Read the model definition and answer for the solid it produces. Units are mm, in the model's axes. A direction names the side the tool comes from. Round coordinates to 2 decimals unless told otherwise and drop trailing zeros. Loops run counter-clockwise (first coordinate to the right, second up) from the corner with the lowest first, then second, coordinate; pieces in that order, holes last. Notation, with made-up numbers: M 37.25,-11.75 L 84.25,-11.75 A22 cw 84.25,6.25 Z; hole C 65,-39.5 d8. An arc over 180 degrees is marked long. Answer as CSV lines item,"result".
```python
from build123d import *

# Parameters (mm, degrees)
SKETCH_1_W          = 60
SKETCH_1_H          = 40
SKETCH_1_R          = 8
EXTRUDE_1_DEPTH     = 3
EXTRUDE_2_DEPTH     = 3
SKETCH_6_W          = 3
SKETCH_6_H          = 68.008301529
EXTRUDE_3_DEPTH     = 60
SKETCH_7_R          = 2.5
CUT_EXTRUDE_1_DEPTH = 121.443081137
FILLET_1_R          = 10
FILLET_2_R          = 20
FILLET_4_R          = 10
FILLET_12_R         = 0.5
FILLET_13_R         = 0.5
SKETCH_10_W         = 25
SKETCH_10_H         = 2.5
EXTRUDE_6_DEPTH     = 75
FILLET_16_R         = 10


with BuildPart() as part:
    # 草图1 → 凸台-拉伸1 (new body)
    with BuildSketch(Plane(origin=(0, 0, 0), x_dir=(1, 0, 0), z_dir=(0, 1, 0))):
        with Locations((-43.647943628, 33.126585816)):
            Rectangle(SKETCH_1_W, SKETCH_1_H)
        with Locations(Location((-33.647943628, 33.126585816, 0), (0, 0, 270))):
            Circle(SKETCH_1_R, mode=Mode.SUBTRACT)
        with BuildLine():
            Line((-18.647943628, 31.626585816), (-22.647943628, 31.626585816))
            ThreePointArc((-22.647943628, 31.626585816), (-24.147943628, 33.126585816), (-22.647943628, 34.626585816))
            Line((-22.647943628, 34.626585816), (-18.647943628, 34.626585816))
            ThreePointArc((-18.647943628, 34.626585816), (-17.147943628, 33.126585816), (-18.647943628, 31.626585816))
        make_face(mode=Mode.SUBTRACT)
        with BuildLine():
            Line((-35.147943628, 18.126585816), (-35.147943628, 22.126585816))
            ThreePointArc((-35.147943628, 22.126585816), (-33.647943628, 23.626585816), (-32.147943628, 22.126585816))
            Line((-32.147943628, 22.126585816), (-32.147943628, 18.126585816))
            ThreePointArc((-32.147943628, 18.126585816), (-33.647943628, 16.626585816), (-35.147943628, 18.126585816))
        make_face(mode=Mode.SUBTRACT)
        with BuildLine():
            Line((-48.647943628, 34.626585816), (-44.647943628, 34.626585816))
            ThreePointArc((-44.647943628, 34.626585816), (-43.147943628, 33.126585816), (-44.647943628, 31.626585816))
            Line((-44.647943628, 31.626585816), (-48.647943628, 31.626585816))
            ThreePointArc((-48.647943628, 31.626585816), (-50.147943628, 33.126585816), (-48.647943628, 34.626585816))
        make_face(mode=Mode.SUBTRACT)
        with BuildLine():
            Line((-32.147943628, 48.126585816), (-32.147943628, 44.126585816))
            ThreePointArc((-32.147943628, 44.126585816), (-33.647943628, 42.626585816), (-35.147943628, 44.126585816))
            Line((-35.147943628, 44.126585816), (-35.147943628, 48.126585816))
            ThreePointArc((-35.147943628, 48.126585816), (-33.647943628, 49.626585816), (-32.147943628, 48.126585816))
        make_face(mode=Mode.SUBTRACT)
        with BuildLine():
            Line((-42.446981734, 20.88620476), (-40.446981734, 24.350306375))
            ThreePointArc((-40.446981734, 24.350306375), (-38.397943628, 24.89934448), (-37.848905522, 22.850306375))
            Line((-37.848905522, 22.850306375), (-39.848905522, 19.38620476))
            ThreePointArc((-39.848905522, 19.38620476), (-41.897943628, 18.837166654), (-42.446981734, 20.88620476))
        make_face(mode=Mode.SUBTRACT)
        with BuildLine():
            Line((-39.848905522, 46.866966873), (-37.848905522, 43.402865258))
            ThreePointArc((-37.848905522, 43.402865258), (-38.397943628, 41.353827152), (-40.446981734, 41.902865258))
            Line((-40.446981734, 41.902865258), (-42.446981734, 45.366966873))
            ThreePointArc((-42.446981734, 45.366966873), (-41.897943628, 47.416004979), (-39.848905522, 46.866966873))
        make_face(mode=Mode.SUBTRACT)
    extrude(amount=EXTRUDE_1_DEPTH)

    # 草图2 → 凸台-拉伸2 (add)
    with BuildSketch(Plane.ZY.offset(73.647943628)):
        Polygon((-67.130736581, 20), (-53.126585816, 0), (-13.126585816, 0), (0.877564948, 20), align=None)
    extrude(amount=EXTRUDE_2_DEPTH)

    # 草图6 → 凸台-拉伸3 (add)
    with BuildSketch(Plane(origin=(0, 20, 0), x_dir=(1, 0, 0), z_dir=(0, 1, 0))):
        with Locations((-75.147943628, 33.126585817)):
            Rectangle(SKETCH_6_W, SKETCH_6_H)
    extrude(amount=EXTRUDE_3_DEPTH)

    # 草图7 → 切除-拉伸1 (cut, through all)
    with BuildSketch(Plane(origin=(-73.647943628, 0, 0), x_dir=(0, 0, -1), z_dir=(1, 0, 0))):
        with Locations((62.130736581, 25)):
            Circle(SKETCH_7_R)
        with Locations((4.130736581, 25)):
            Circle(SKETCH_7_R)
        with Locations((62.130736581, 70)):
            Circle(SKETCH_7_R)
        with Locations((4.130736581, 70)):
            Circle(SKETCH_7_R)
    extrude(amount=-CUT_EXTRUDE_1_DEPTH, mode=Mode.SUBTRACT)

    # 圆角1
    fillet_1_edges = [part.edges().sort_by_distance(p)[0] for p in [
        (-13.647943628, 1.5, -53.126585816),
        (-13.647943628, 1.5, -13.126585816),
    ]]
    fillet(fillet_1_edges, radius=FILLET_1_R)

    # 圆角2
    fillet_2_edges = [part.edges().sort_by_distance(p)[0] for p in [
        (-75.147943628, 20, 0.877564948),
        (-75.147943628, 20, -67.130736581),
    ]]
    fillet(fillet_2_edges, radius=FILLET_2_R)

    # 圆角4
    fillet_4_edges = [part.edges().sort_by_distance(p)[0] for p in [
        (-75.147943628, 80, -67.130736581),
        (-75.147943628, 80, 0.877564948),
    ]]
    fillet(fillet_4_edges, radius=FILLET_4_R)

    # 圆角12
    fillet_12_edges = [part.edges().sort_by_distance(p)[0] for p in [
        (-73.647943628, 7.417223525, -7.932989991),
        (-73.647943628, 7.417223525, -58.320181641),
        (-73.647943628, 20.291859787, -0.048096037),
        (-73.647943628, 20.291859787, -66.205075596),
        (-73.647943628, 80, -33.126585816),
        (-73.647943628, 48.152987889, -67.130736581),
        (-73.647943628, 48.152987889, 0.877564948),
        (-73.647943628, 77.071067812, -64.201804393),
        (-73.647943628, 77.071067812, -2.05136724),
    ]]
    fillet(fillet_12_edges, radius=FILLET_12_R)

    # 圆角13
    fillet_13_edges = [part.edges().sort_by_distance(p)[0] for p in [
        (-76.647943628, 7.417223525, -7.932989991),
        (-76.647943628, 7.417223525, -58.320181641),
        (-76.647943628, 20.291859787, -0.048096037),
        (-76.647943628, 20.291859787, -66.205075596),
        (-76.647943628, 80, -33.126585816),
        (-76.647943628, 48.152987889, 0.877564948),
        (-76.647943628, 48.152987889, -67.130736581),
        (-76.647943628, 77.071067812, -64.201804393),
        (-76.647943628, 77.071067812, -2.05136724),
    ]]
    fillet(fillet_13_edges, radius=FILLET_13_R)

    # 草图10 → 凸台-拉伸6 (add)
    with BuildSketch(Plane(origin=(0, 3, 0), x_dir=(1, 0, 0), z_dir=(0, 1, 0))):
        with Locations((-61.147943628, 51.876585816)):
            Rectangle(SKETCH_10_W, SKETCH_10_H)
        with Locations((-61.147943628, 14.376585816)):
            Rectangle(SKETCH_10_W, SKETCH_10_H)
    extrude(amount=EXTRUDE_6_DEPTH)

    # 圆角16
    fillet_16_edges = [part.edges().sort_by_distance(p)[0] for p in [
        (-48.647943628, 78, -51.876585816),
        (-48.647943628, 78, -14.376585816),
    ]]
    fillet(fillet_16_edges, radius=FILLET_16_R)


solid = part.part
```
1) A tool of negligible diameter and unlimited length cuts with its end or side. For faces 4 (the flat face through (-61, 40, -15.627)), 5 (the flat face through (-13.648, 1, -33)), 6 (the flat face through (-47, 1, -34.627)), 7 (the flat face through (-48.648, 35, -52)), 8 (the cylindrical face through (-16.5, 1.52, -50.12)), from which of +Z, -Z, +X, -X, +Y, -Y can it reach the whole face along a straight path? Write none if from no direction.
Evaluation:
face 4,"+X, +Y"
face 5,"+Z, -Z, +X, +Y, -Y"
face 6,"+Y, -Y"
face 7,"+Z, -Z, +X, +Y"
face 8,"-Z, +X, +Y, -Y"
2) Straight lines are drawn through the part: line 1 (Z direction, x = -58.5, y = 11); line 2 (X direction, y = 64, z = -52.5); line 3 (Y direction, x = -42.5, z = -31). For each, find the intervals that lie inside material, in ascending order.
Evaluation:
line 1,"z = -53.13 to -50.63, -15.63 to -13.13"
line 2,"x = -76.65 to -48.65"
line 3,"y = 0 to 3"
3) Find section C-C, the plane y = 56.5. Give the vertices of the cut face in (x, z), then the cut area to 3 significant figures.
Evaluation:
outline,"M -76.65,-66.63 A0.5 ccw -76.15,-67.13 L -74.15,-67.13 A0.5 ccw -73.65,-66.63 L -73.65,-53.13 L -48.65,-53.13 L -48.65,-50.63 L -73.65,-50.63 L -73.65,-15.63 L -48.65,-15.63 L -48.65,-13.13 L -73.65,-13.13 L -73.65,0.38 A0.5 ccw -74.15,0.88 L -76.15,0.88 A0.5 ccw -76.65,0.38 Z"
area,"329 mm^2"
4) Determine the mould class of faces 1 (the cylindrical face through (-16.655, 1.521, -15.978)), 2 (the cylindrical face through (-17.15, 1.48, -33.16)), 3 (the flat face through (-75, 80, -33)) for opening direction Z: released by +Z, released by -Z, zero draft, split by the parting line, or undercut.
Evaluation:
face 1,"released by +Z"
face 2,"undercut"
face 3,"zero draft"
5) Find section D-D, the plane y = 25. Count the separate pieces of the cut face and the enclosed holes in it, then the cut area to 3 significant figures.
Evaluation:
separate pieces,"3"
enclosed holes,"0"
area,"299 mm^2"
6) Find section B-B, the plane x = -68. Give the vertices of the cut face in (y, z), then the cut area to 3 significant figures.
Evaluation:
outline,"M 0,-53.13 L 78,-53.13 L 78,-50.63 L 3,-50.63 L 3,-15.63 L 78,-15.63 L 78,-13.13 L 0,-13.13 Z"
area,"495 mm^2"
7) Find section A-A, the plane z = -36. Give the vertices of the cut face in (x, y), then the cut area to 3 significant figures.
Evaluation:
outline,"M -76.65,0 L -41.11,0 L -41.11,3 L -73.65,3 L -73.65,79.5 A0.5 ccw -74.15,80 L -76.15,80 A0.5 ccw -76.65,79.5 Z; M -26.18,0 L -13.65,0 L -13.65,3 L -26.18,3 Z"
area,"375 mm^2"
8) Each of these flat-tipped pins is pushed along its axis until it touches: P1, Ø12.5, axis at x = -60, y = 35.5, coming from the +Z side; P2, Ø8, axis at x = -27, z = -26.5, coming from the +Y side; P3, Ø2.5, axis at x = -20.5, y = 1, coming from the -Z side. Where does it stop, or does it pass through?
Evaluation:
P1,"stops at z = -13.13"
P2,"stops at y = 3"
P3,"stops at z = -52.94"
